CAD build for the part. Positions are in the model's coordinates, mm. Face numbers are marked on the shaded views. Give positions to 0.01 mm unless a question says otherwise; leave off trailing zeros. Order: outer loops, then holes, each group sorted by start corner. A loop starts at its lowest first (then second) coordinate and runs counter-clockwise, first axis right, second up.
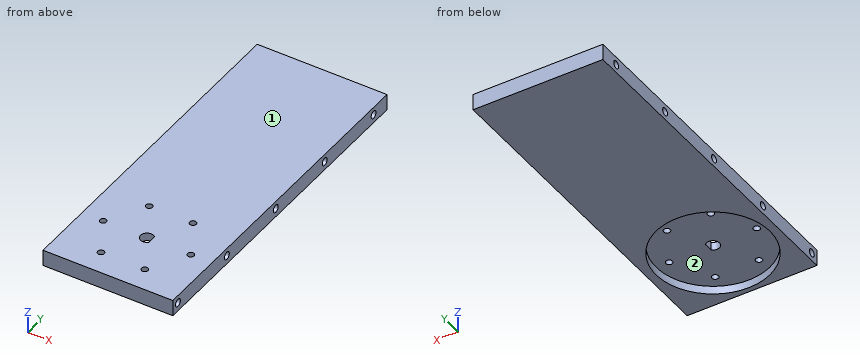
```python
from build123d import *

# Parameters (mm, degrees)
CROQUIS1_W              = 80
CROQUIS1_H              = 200
SALIENTE_EXTRUIR1_DEPTH = 10
CORTAR_EXTRUIR1_DEPTH   = 10
CROQUIS5_R              = 2
CORTAR_EXTRUIR4_DEPTH   = 216.638586528
CROQUIS6_R              = 35
CORTAR_EXTRUIR5_DEPTH   = 5
CROQUIS7_W              = 80
CROQUIS7_H              = 8
SALIENTE_EXTRUIR2_DEPTH = 10
CROQUIS9_R              = 35
CORTAR_EXTRUIR7_DEPTH   = 5
CROQUIS11_R             = 2.35
CORTAR_EXTRUIR8_DEPTH   = 5
CROQUIS12_R             = 2.35
CORTAR_EXTRUIR9_DEPTH   = 5


with BuildPart() as part:
    # Croquis1 → Saliente-Extruir1 (new body)
    with BuildSketch(Plane.XY):
        with Locations((40, 100)):
            Rectangle(CROQUIS1_W, CROQUIS1_H)
    extrude(amount=SALIENTE_EXTRUIR1_DEPTH)

    # Croquis2 → Cortar-Extruir1 (cut)
    with BuildSketch(Plane.XY.offset(10)):
        with BuildLine():
            Line((42.90473751, 27.25), (42.90473751, 32.75))
            ThreePointArc((42.90473751, 32.75), (36, 30), (42.90473751, 27.25))
        make_face()
    extrude(amount=-CORTAR_EXTRUIR1_DEPTH, mode=Mode.SUBTRACT)

    # Croquis5 → Cortar-Extruir4 (cut, through all)
    with BuildSketch(Plane(origin=(0, 0, 0), x_dir=(-1, 0, 0), z_dir=(0, 0, -1))):
        with Locations((-13, 30)):
            Circle(CROQUIS5_R)
        with Locations((-26.5, 6.617314098)):
            Circle(CROQUIS5_R)
        with Locations((-53.5, 6.617314098)):
            Circle(CROQUIS5_R)
        with Locations((-67, 30)):
            Circle(CROQUIS5_R)
        with Locations((-53.5, 53.382685902)):
            Circle(CROQUIS5_R)
        with Locations((-26.5, 53.382685902)):
            Circle(CROQUIS5_R)
    extrude(amount=-CORTAR_EXTRUIR4_DEPTH, mode=Mode.SUBTRACT)

    # Croquis6 → Cortar-Extruir5 (cut)
    with BuildSketch(Plane(origin=(0, 0, 0), x_dir=(-1, 0, 0), z_dir=(0, 0, -1))):
        with Locations((-40, 30)):
            Circle(CROQUIS6_R)
    extrude(amount=-CORTAR_EXTRUIR5_DEPTH, mode=Mode.SUBTRACT)

    # Croquis7 → Saliente-Extruir2 (add)
    with BuildSketch(Plane.XY.offset(10)):
        with Locations((40, -4)):
            Rectangle(CROQUIS7_W, CROQUIS7_H)
    extrude(amount=-SALIENTE_EXTRUIR2_DEPTH)

    # Croquis9 → Cortar-Extruir7 (cut)
    with BuildSketch(Plane(origin=(0, 0, 0), x_dir=(-1, 0, 0), z_dir=(0, 0, -1))):
        with Locations((-40, 30)):
            Circle(CROQUIS9_R)
    extrude(amount=-CORTAR_EXTRUIR7_DEPTH, mode=Mode.SUBTRACT)

    # Croquis11 → Cortar-Extruir8 (cut)
    with BuildSketch(Plane.ZY):
        with Locations(Location((5, 187, 0), (0, 0, 270))):
            Circle(CROQUIS11_R)
        with Locations(Location((5, 139.5, 0), (0, 0, 270))):
            Circle(CROQUIS11_R)
        with Locations(Location((5, 92, 0), (0, 0, 270))):
            Circle(CROQUIS11_R)
        with Locations(Location((5, 44.5, 0), (0, 0, 270))):
            Circle(CROQUIS11_R)
        with Locations(Location((5, -3, 0), (0, 0, 270))):
            Circle(CROQUIS11_R)
    extrude(amount=-CORTAR_EXTRUIR8_DEPTH, mode=Mode.SUBTRACT)

    # Croquis12 → Cortar-Extruir9 (cut)
    with BuildSketch(Plane(origin=(80, 0, 0), x_dir=(0, 0, -1), z_dir=(1, 0, 0))):
        with Locations(Location((-5.28576423, 187, 0), (0, 0, 90))):
            Circle(CROQUIS12_R)
        with Locations(Location((-5.28576423, 139.5, 0), (0, 0, 90))):
            Circle(CROQUIS12_R)
        with Locations(Location((-5.28576423, 92, 0), (0, 0, 90))):
            Circle(CROQUIS12_R)
        with Locations(Location((-5.28576423, 44.5, 0), (0, 0, 90))):
            Circle(CROQUIS12_R)
        with Locations(Location((-5.28576423, -3, 0), (0, 0, 90))):
            Circle(CROQUIS12_R)
    extrude(amount=-CORTAR_EXTRUIR9_DEPTH, mode=Mode.SUBTRACT)


solid = part.part
```
Item 1: Drop flat-ended pins along their axis: pin 1 Ø1.4 at (y, z) = (140, 5.5) entering from -X; pin 2 Ø3 at (x, y) = (53.5, 6.62) entering from +Z; pin 3 Ø2.5 at (y, z) = (92, 4.5) entering from +X. Give the stop position or say it passes through.
Item 2: Wall check: L1, parallel to Y at x = 53.5, z = 6.45; L2, parallel to Z at x = 78.55, y = 187; L3, parallel to Y at x = 40, z = 1.35. Give the ranges that are in metal, low to high.
Item 3: Slice it at B-B (x = 53.5). Give the cut face in (y, z), and give its area (3 significant figures).
Item 4: Slice it at C-C (y = 92). Give the cut face in (x, z), and give its area (3 significant figures).
Item 5: Two-plate mould, pull along X, no slides. Class the marked faces 1 and 2: released by +X, released by -X, zero draft, split by the parting line, or undercut.
Item 6: Slice it at A-A (x = 40). Give the cut face in (y, z).
Item 7: Slice it at D-D (x = 67). Give the cut face in (y, z), and give its area (3 significant figures).
A:
1. pin 1: stops at x = 5
1. pin 2: passes through
1. pin 3: stops at x = 75
2. L1: y = -8 to 4.62, 8.62 to 51.38, 55.38 to 200
2. L2: z = 0 to 2.94, 7.64 to 10
2. L3: y = -8 to -5, 65 to 200
3. outline: (-8, 0) - (-2.29, 0) - (-2.29, 5) - (4.62, 5) - (4.62, 10) - (-8, 10) - close; (8.62, 5) - (51.38, 5) - (51.38, 10) - (8.62, 10) - close; (55.38, 5) - (62.29, 5) - (62.29, 0) - (200, 0) - (200, 10) - (55.38, 10) - close
3. area: 1,720 mm2
4. outline: (0, 0) - (80, 0) - (80, 2.94) - (75, 2.94) - (75, 7.64) - (80, 7.64) - (80, 10) - (0, 10) - (0, 7.35) - (5, 7.35) - (5, 2.65) - (0, 2.65) - close
4. area: 753 mm2
5. face 1: zero draft
5. face 2: undercut
6. outline: (-8, 0) - (-5, 0) - (-5, 5) - (26, 5) - (26, 10) - (-8, 10) - close; (34, 5) - (65, 5) - (65, 0) - (200, 0) - (200, 10) - (34, 10) - close
7. outline: (-8, 0) - (7.73, 0) - (7.73, 5) - (28, 5) - (28, 10) - (-8, 10) - close; (32, 5) - (52.27, 5) - (52.27, 0) - (200, 0) - (200, 10) - (32, 10) - close
7. area: 1,840 mm2
